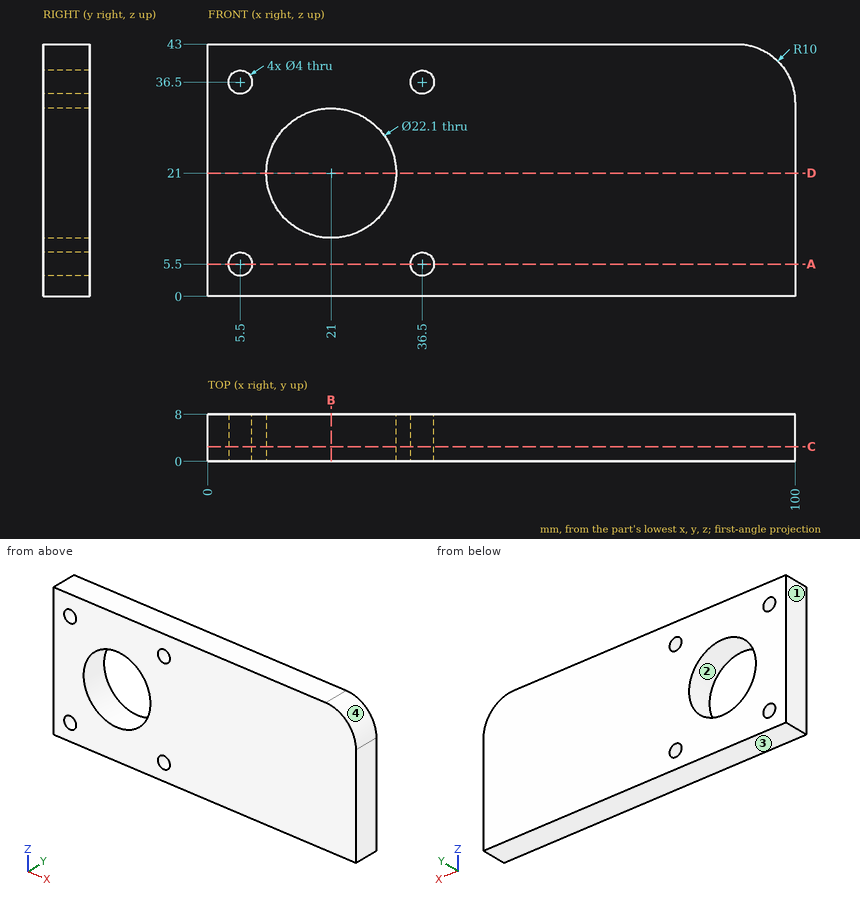
Could you check a few things on this drawing? It's one solid part, dimensions in mm from its lowest x, y, z. Give positions to 0.01 mm unless a question says otherwise; leave off trailing zeros. Order: outer loops, then holes, each group sorted by start corner. A loop starts at its lowest first (then second) coordinate and runs counter-clockwise, first axis right, second up. Notation, with made-up numbers: (21.5, -3.75) - (57.5, -3.75) arc R33 ccw to (57.5, 29.25) - close; hole circle Ø4 at (36.5, -35). An arc over 180 degrees is marked (long way). One line per question, with ' | ' between items. Start each with the question number.
Item 1: I want a section at B-B on x = 21. Write out the boundary of the cut face in (y, z), then the cut area to 3 significant figures.
Item 2: I want a section at C-C on y = 2.5. Write out the boundary of the cut face in (x, z).
Item 3: Thinking about a two-plate mould opening in X: for the marked faces 1, 2, 3 and 4, which applies, pulls with the +X half, pulls with the -X half, needs draft (parallel to the pull), parting line crosses it, or undercut?
Item 4: I want a section at D-D on z = 21. Write out the boundary of the cut face in (x, y).
Item 5: I need wall thicknesses on probe 1 along Z at (x, y) = (36.5, 6); probe 2 along X at (y, z) = (4.25, 5.5); probe 3 along X at (y, z) = (4, 36.5). Which ranges of each line are inside material? Lowest first, please. Write a range as [from, to].
Item 6: I want a section at A-A on z = 5.5. Write out the boundary of the cut face in (x, y), then the cut area to 3 significant figures.
Verdict:
1) outline: (0, 0) - (8, 0) - (8, 9.95) - (0, 9.95) - close; (0, 32.05) - (8, 32.05) - (8, 43) - (0, 43) - close | area: 167 mm^2
2) outline: (0, 0) - (100, 0) - (100, 33) arc R10 ccw to (90, 43) - (0, 43) - close; hole circle Ø4 at (5.5, 5.5); hole circle Ø4 at (5.5, 36.5); hole circle Ø22.1 at (21, 21); hole circle Ø4 at (36.5, 5.5); hole circle Ø4 at (36.5, 36.5)
3) face 1: pulls with the -X half | face 2: undercut | face 3: needs draft | face 4: pulls with the +X half
4) outline: (0, 0) - (9.95, 0) - (9.95, 8) - (0, 8) - close; (32.05, 0) - (100, 0) - (100, 8) - (32.05, 8) - close
5) probe 1: [0, 3.5], [7.5, 34.5], [38.5, 43] | probe 2: [0, 3.5], [7.5, 34.5], [38.5, 100] | probe 3: [0, 3.5], [7.5, 34.5], [38.5, 99.37]
6) outline: (0, 0) - (3.5, 0) - (3.5, 8) - (0, 8) - close; (7.5, 0) - (34.5, 0) - (34.5, 8) - (7.5, 8) - close; (38.5, 0) - (100, 0) - (100, 8) - (38.5, 8) - close | area: 736 mm^2
